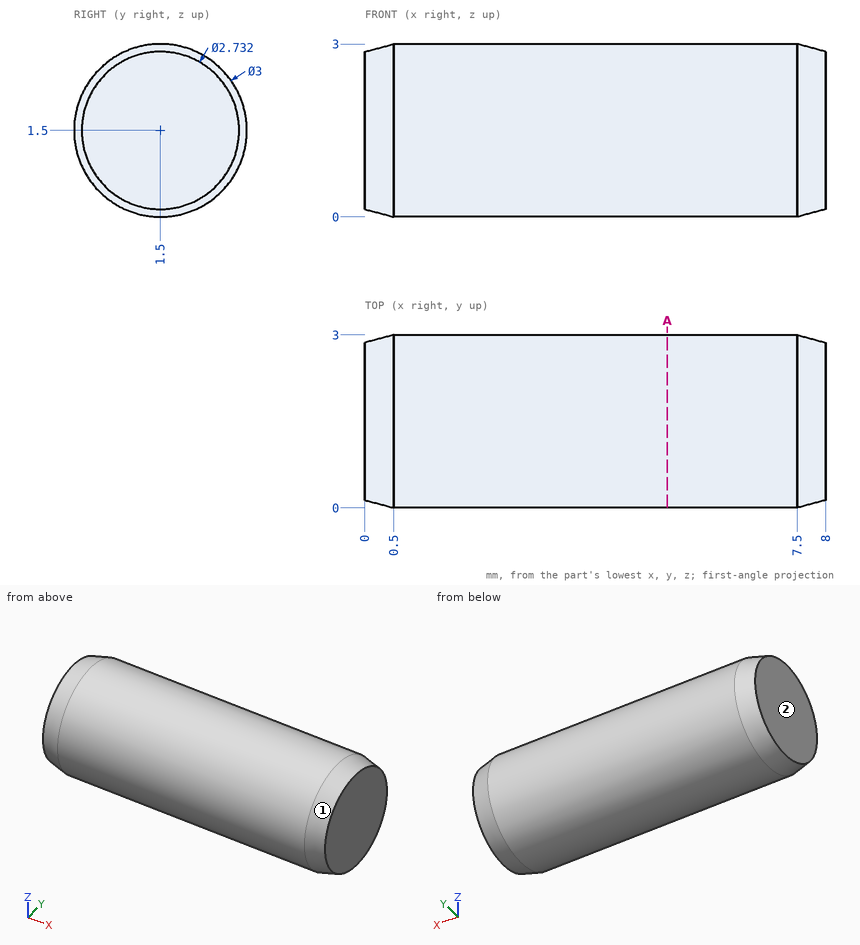
Can you work these out from the drawing? Everything is in mm from the part's minimum corner. Round coordinates to 2 decimals unless told otherwise and drop trailing zeros. Loops run counter-clockwise (first coordinate to the right, second up) from the corner with the lowest first, then second, coordinate; pieces in that order, holes last. Notation, with made-up numbers: (-9, 5.5) - (1, 5.5) arc R21 cw to (1, 23.5) - close; hole circle Ø2 at (28, 50). An arc over 180 degrees is marked (long way). Answer in a Markdown table with one row per item. Add a question column.
(1) If we section it at A-A (x = 5.25): Please give me the cut outline in (y, z), plus the area to 3 significant figures.
(2) If we mould it in two halves opening along Y, with no side actions, what happens to the marked faces 1 and 2? For each: pulls with the +Y half, pulls with the -Y half, needs draft (parallel to the pull), parting line crosses it, or undercut.
(3) I need wall thicknesses on line 1 along Y through (x, z) = (5.75, 0.85); line 2 along Z through (x, y) = (2.25, 2.4); line 3 along Z through (x, y) = (4.75, 2.7). Which ranges of each line are inside material? Lowest first, please.
(4) I'm going to push a flat-ended pin straight in: pin 1 (1.5 mm diameter, centred on x = 3, z = 0.5, fed in from -Y). Where does the tip first touch, or does it pass through?
Model answer:
| question | item | result |
|---|---|---|
| 1 | outline | circle Ø3 at (1.5, 1.5) |
| 1 | area | 7.07 mm² |
| 2 | face 1 | parting line crosses it |
| 2 | face 2 | needs draft |
| 3 | line 1 | y = 0.15 to 2.85 |
| 3 | line 2 | z = 0.3 to 2.7 |
| 3 | line 3 | z = 0.6 to 2.4 |
| 4 | pin 1 | stops at y = 0.02 |
